Could you check a few things on this model? Use its own coordinates, in mm. Face numbers are marked on the shaded views. A direction names the side the tool comes from. Give positions to 0.01 mm unless a question says otherwise; leave off trailing zeros. Loops run counter-clockwise (first coordinate to the right, second up) from the corner with the lowest first, then second, coordinate; pieces in that order, holes last. Notation, with made-up numbers: (-5, -3) - (3, -3) arc R24 cw to (3, 32) - close; hole circle Ø11 at (-40, -4.75). An arc over 180 degrees is marked (long way). Write each question's results on one line, items separated by ' | '. Start each with the question number.
(1) If we mould it in two halves opening along X, with no side actions, what happens to the marked faces 3, 4 and 5? For each: released by +X, released by -X, zero draft, split by the parting line, or undercut.
(2) Suppose I cut it at B-B (z = -23). Please give me the cut outline in (x, y).
(3) For pin 1 (5 mm diameter, centred on x = -15.5, z = -22.5, fed in from -Y); pin 2 (1.5 mm diameter, centred on x = -21.5, z = -3.5, fed in from +Y); pin 3 (4 mm diameter, centred on x = -15.5, y = 5.5, fed in from -Z); pin 4 (1 mm diameter, centred on y = 7, z = -12.5, fed in from -X), each with a flat end and sliding along its axis, tell me the tip position at first contact or that it passes through.
(4) On a 3-axis mill with a long thin cutter (end or side, diameter ignored), from which of +Z, -Z, +X, -X, +Y, -Y can I reach the whole of each face in a straight line? I mean the marked faces 1 and 2. Say none if no direction works.
(5) Suppose I cut it at D-D (x = -33.5). Please give me the cut outline in (y, z), and give its area (3 significant figures).
(6) Suppose I cut it at A-A (y = 5.5). Count the separate pieces of the cut face and the enclosed holes in it, and give its area (3 significant figures).
(7) I need wall thicknesses on line 1 (Z direction, x = -21, y = 8); line 2 (X direction, y = 5.5, z = -12.5); line 3 (Y direction, x = -15.5, z = -14). Which ranges of each line are inside material? Lowest first, please.
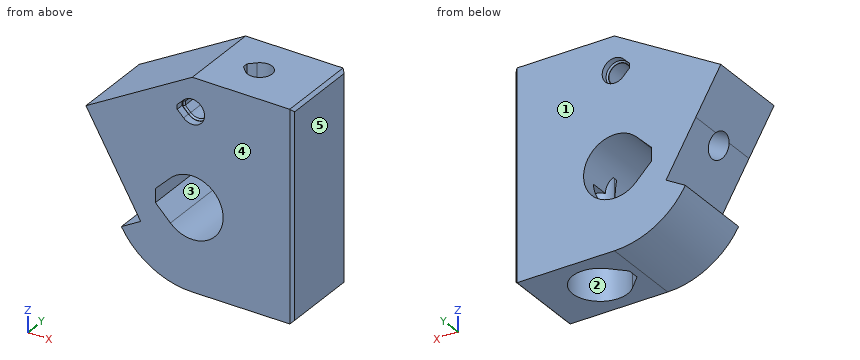
from build123d import *

# Parameters (mm, degrees)
SKETCH1_R           = 4.15
BOSS_EXTRUDE1_DEPTH = 11
SKETCH2_R           = 1.65
CUT_EXTRUDE1_DEPTH  = 29
SKETCH3_R           = 3.7
CUT_EXTRUDE2_DEPTH  = 11
SKETCH5_R           = 1.4
CUT_EXTRUDE4_DEPTH  = 12.0000001
SKETCH11_R          = 1.4
CUT_EXTRUDE10_DEPTH = 14
CUT_EXTRUDE14_DEPTH = 12.0000001
CUT_EXTRUDE15_DEPTH = 11
CUT_EXTRUDE16_DEPTH = 29.0000001
CUT_EXTRUDE21_DEPTH = 12.0000001
SKETCH20_R          = 1.65
CUT_EXTRUDE18_DEPTH = 1
SKETCH21_R          = 1.65
CUT_EXTRUDE19_DEPTH = 1
CUT_EXTRUDE22_DEPTH = 1
CUT_EXTRUDE23_DEPTH = 1
CHAMFER4_SIZE       = 0.4
CUT_EXTRUDE20_DEPTH = 9
CHAMFER5_SIZE       = 0.2


with BuildPart() as part:
    # Sketch1 → Boss-Extrude1 (new body)
    with BuildSketch(Plane(origin=(0, 0, 0), x_dir=(1, 0, 0), z_dir=(0, 1, 0))):
        with BuildLine():
            Line((-7.5, -1), (-21, -1))
            Line((-21, -1), (-35.289419162, 7.25))
            Line((-35.289419162, 7.25), (-31.92820323, 13.07179677))
            Line((-31.92820323, 13.07179677), (-27.92820323, 20))
            Line((-27.92820323, 20), (-30.526279442, 21.5))
            ThreePointArc((-30.526279442, 21.5), (-26.5, 25.526279442), (-21, 27))
            Line((-21, 27), (-7.5, 27))
            Line((-7.5, 27), (-7.5, -1))
        make_face()
        with Locations((-21, 16)):
            Circle(SKETCH1_R, mode=Mode.SUBTRACT)
    extrude(amount=BOSS_EXTRUDE1_DEPTH)

    # Sketch2 → Cut-Extrude1 (cut, through all)
    with BuildSketch(Plane.XY.offset(1)):
        with Locations((-15.5, 5.5)):
            Circle(SKETCH2_R)
    extrude(amount=-CUT_EXTRUDE1_DEPTH, mode=Mode.SUBTRACT)

    # Sketch3 → Cut-Extrude2 (cut)
    with BuildSketch(Plane(origin=(0, 0, -27), x_dir=(-1, 0, 0), z_dir=(0, 0, -1))):
        with Locations((15.5, 5.5)):
            Circle(SKETCH3_R)
    extrude(amount=-CUT_EXTRUDE2_DEPTH, mode=Mode.SUBTRACT)

    # Sketch5 → Cut-Extrude4 (cut, through all)
    with BuildSketch(Plane(origin=(0, 11, 0), x_dir=(1, 0, 0), z_dir=(0, 1, 0))):
        with Locations((-21, 3.5)):
            Circle(SKETCH5_R)
    extrude(amount=-CUT_EXTRUDE4_DEPTH, mode=Mode.SUBTRACT)

    # Sketch11 → Cut-Extrude10 (cut)
    with BuildSketch(Plane(origin=(-29.606406461, 0, -17.09326674), x_dir=(-0.5, 0, 0.866025404), z_dir=(-0.866025404, 0, -0.5))):
        with Locations((3.643593539, 5.5)):
            Circle(SKETCH11_R)
    extrude(amount=-CUT_EXTRUDE10_DEPTH, mode=Mode.SUBTRACT)

    # Sketch16 → Cut-Extrude14 (cut, through all)
    with BuildSketch(Plane.XZ):
        Polygon((-21, -16), (-23.934493142, -18.934493142), (-25.95, -16.918986284), (-25.95, -15.081013716), (-23.934493142, -13.065506858), align=None)
    extrude(amount=-CUT_EXTRUDE14_DEPTH, mode=Mode.SUBTRACT)

    # Sketch17 → Cut-Extrude15 (cut)
    with BuildSketch(Plane(origin=(0, 0, -27), x_dir=(-1, 0, 0), z_dir=(0, 0, -1))):
        Polygon((15.5, 5.5), (18.11629509, 2.88370491), (19.94, 4.707409819), (19.94, 6.292590181), (18.11629509, 8.11629509), align=None)
    extrude(amount=-CUT_EXTRUDE15_DEPTH, mode=Mode.SUBTRACT)

    # Sketch18 → Cut-Extrude16 (cut, through all)
    with BuildSketch(Plane.XY.offset(1)):
        Polygon((-15.5, 5.5), (-16.666726189, 6.666726189), (-17.47, 5.863452378), (-17.47, 5.136547622), (-16.666726189, 4.333273811), align=None)
    extrude(amount=-CUT_EXTRUDE16_DEPTH, mode=Mode.SUBTRACT)

    # Sketch23 → Cut-Extrude21 (cut, through all)
    with BuildSketch(Plane.XZ):
        Polygon((-21.989949494, -2.510050506), (-22.72, -3.240101013), (-22.72, -3.759898987), (-21.989949494, -4.489949494), align=None)
    extrude(amount=-CUT_EXTRUDE21_DEPTH, mode=Mode.SUBTRACT)

    # Sketch20 → Cut-Extrude18 (cut)
    with BuildSketch(Plane(origin=(0, 11, 0), x_dir=(1, 0, 0), z_dir=(0, 1, 0))):
        with Locations((-21, 3.5)):
            Circle(SKETCH20_R)
    extrude(amount=-CUT_EXTRUDE18_DEPTH, mode=Mode.SUBTRACT)

    # Sketch21 → Cut-Extrude19 (cut)
    with BuildSketch(Plane.XZ):
        with Locations((-21, -3.5)):
            Circle(SKETCH21_R)
    extrude(amount=-CUT_EXTRUDE19_DEPTH, mode=Mode.SUBTRACT)

    # Sketch24 → Cut-Extrude22 (cut)
    with BuildSketch(Plane.XZ):
        Polygon((-22.166726189, -2.333273811), (-23.02, -3.186547622), (-23.02, -3.813452378), (-22.166726189, -4.666726189), align=None)
    extrude(amount=-CUT_EXTRUDE22_DEPTH, mode=Mode.SUBTRACT)

    # Sketch25 → Cut-Extrude23 (cut)
    with BuildSketch(Plane(origin=(0, 11, 0), x_dir=(1, 0, 0), z_dir=(0, 1, 0))):
        Polygon((-23.02, 3.186547622), (-23.02, 3.813452378), (-22.166726189, 4.666726189), (-22.166726189, 2.333273811), align=None)
    extrude(amount=-CUT_EXTRUDE23_DEPTH, mode=Mode.SUBTRACT)

    # Chamfer4
    chamfer4_edges = [part.edges().sort_by_distance(p)[0] for p in [
        (-7.5, 11, -13),
        (-7.5, 5.5, -27),
        (-7.5, 5.5, 1),
        (-7.5, 0, -13),
    ]]
    chamfer(chamfer4_edges, length=CHAMFER4_SIZE)

    # Sketch22 → Cut-Extrude20 (cut)
    with BuildSketch(Plane(origin=(-29.606406461, 0, -17.09326674), x_dir=(-0.5, 0, 0.866025404), z_dir=(-0.866025404, 0, -0.5))):
        with BuildLine():
            ThreePointArc((2.441512011, 6.702081528), (3.643593539, 3.8), (4.845675067, 6.702081528))
            ThreePointArc((4.845675067, 6.702081528), (3.643593539, 7.2), (2.441512011, 6.702081528))
        make_face()
    extrude(amount=-CUT_EXTRUDE20_DEPTH, mode=Mode.SUBTRACT)

    # Chamfer5
    chamfer5_edges = [part.edges().sort_by_distance(p)[0] for p in [
        (-22.354974747, 1, -2.87507576),
        (-19.6, 1, -3.5),
        (-22.354974747, 1, -4.12492424),
        (-22.72, 1, -3.5),
        (-19.35, 10, -3.5),
        (-22.593363094, 10, -2.759910717),
        (-22.593363094, 10, -4.240089283),
        (-22.72, 10, -3.5),
    ]]
    chamfer(chamfer5_edges, length=CHAMFER5_SIZE)


solid = part.part
Output values:
1) face 3: undercut | face 4: zero draft | face 5: released by +X
2) outline: (-29.49, 0) - (-7.9, 0) - (-7.5, 0.4) - (-7.5, 10.6) - (-7.9, 11) - (-29.49, 11) - close; hole (-19.94, 4.71) - (-18.12, 2.88) arc R3.7 ccw (long way) to (-18.12, 8.12) - (-19.94, 6.29) - close
3) pin 1: y = 0 | pin 2: through | pin 3: z = -16 | pin 4: x = -32.55
4) face 1: +Z, -Z, +X, -X, +Y | face 2: -Z
5) outline: (0, -10.35) - (11, -10.35) - (11, -6.22) - (0, -6.22) - close | area: 45.5 mm2
6) separate pieces: 2 | enclosed holes: 1 | area: 372 mm2
7) line 1: -27 to -20.15, -11.85 to -4.9, -2.1 to 1 | line 2: -25.54 to -23.23, -18.77 to -17.47, -13.85 to -7.5 | line 3: 0 to 3.85, 7.15 to 11
